Here's the drawing with two shaded views (mm, measured from the low corner). I have some questions. A direction names the side the tool comes from. Give positions to 0.01 mm unless a question says otherwise; leave off trailing zeros. Write each loop counter-clockwise with the first axis right and the second up, starting at its lowest first coordinate (ties: lowest second). Pieces come first, ordered by that corner, then holes.
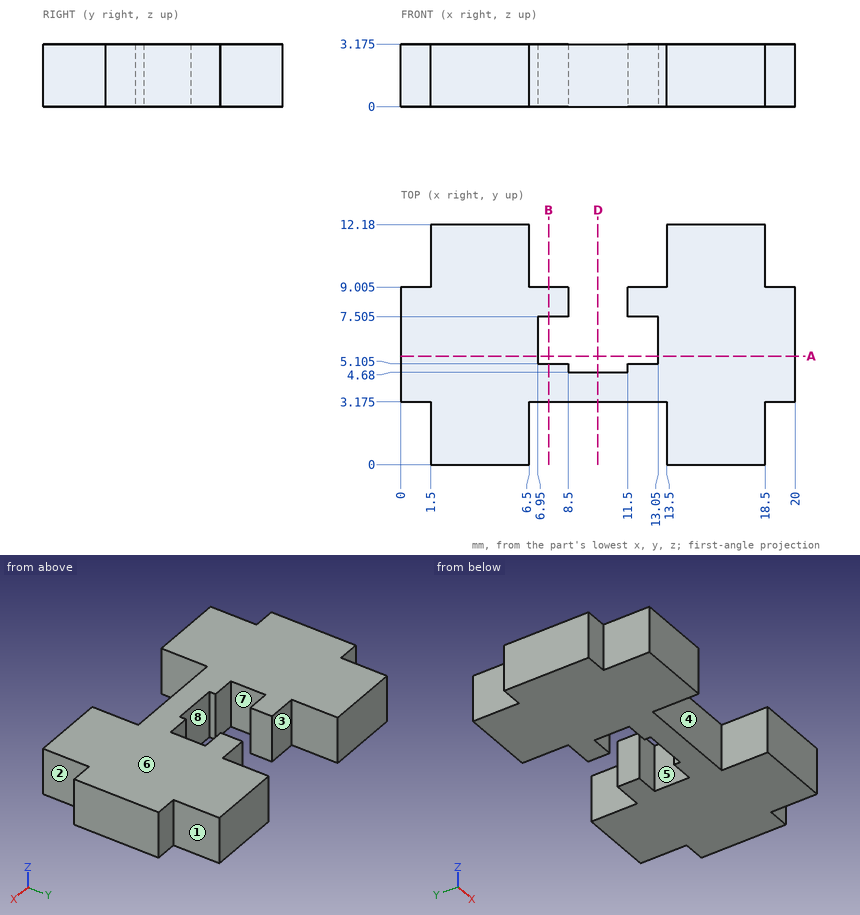
(1) If we mould it in two halves opening along Y, with no side actions, what happens to the marked faces 5, 6, 7 and 8? For each: +Y half, -Y half, draft (parallel to the pull), parting line (faces both ways), or undercut.
Returned:
face 5: undercut
face 6: draft
face 7: undercut
face 8: +Y half
(2) If I drill on L1, parallel to X at y = 2.25, z = 1.45; L2, parallel to X at y = 6.5, z = 0.7; L3, parallel to Y at x = 7, z = 1.3 (3 decimals), over which ranges is the centre line in solid material (lowest first)?
Returned:
L1: x = 1.5 to 6.5, 13.5 to 18.5
L2: x = 0 to 6.95, 13.05 to 20
L3: y = 3.175 to 5.105, 7.505 to 9.005
(3) For the marked faces 1, 2, 3 and 4, which set-ups out of +Z, -Z, +X, -X, +Y, -Y let a thin tool reach every point of the face, with its end or its side?
Returned:
face 1: +Z, -Z, +X, +Y
face 2: +Z, -Z, +X, -Y
face 3: +Z, -Z, +Y
face 4: +Z, -Z, -Y
(4) Will these pins go through, and if not, where does the flat tip stop? P1, Ø1.7, axis at x = 7.5, z = 2, coming from the -Y side (3 decimals); P2, Ø1.6, axis at y = 1, z = 2, coming from the +X side; P3, Ø1, axis at y = 1, z = 2, coming from the -X side; P4, Ø4, axis at x = 4.5, y = 6, coming from the -Z side.
Returned:
P1: stops at y = 3.175
P2: stops at x = 18.5
P3: stops at x = 1.5
P4: stops at z = 0
(5) Imagine slicing it at A-A, the plane y = 5.5. Write out the boundary of the cut face in (x, z) (3 decimals), plus the area to 3 significant figures.
Returned:
outline: (0, 0) - (6.95, 0) - (6.95, 3.175) - (0, 3.175) - close; (13.05, 0) - (20, 0) - (20, 3.175) - (13.05, 3.175) - close
area: 44.1 mm2
(6) Imagine slicing it at B-B, the plane x = 7.5. Write out the boundary of the cut face in (y, z) (3 decimals), plus the area to 3 significant figures.
Returned:
outline: (3.175, 0) - (5.105, 0) - (5.105, 3.175) - (3.175, 3.175) - close; (7.505, 0) - (9.005, 0) - (9.005, 3.175) - (7.505, 3.175) - close
area: 10.9 mm2
(7) Imagine slicing it at D-D, the plane x = 10. Write out the boundary of the cut face in (y, z) (3 decimals), plus the area to 3 significant figures.
Returned:
outline: (3.175, 0) - (4.68, 0) - (4.68, 3.175) - (3.175, 3.175) - close
area: 4.78 mm2
